Here's how the part is built. I have some questions about the finished solid (model axes, mm). A direction names the side the tool comes from. Give positions to 0.01 mm unless a question says otherwise; leave off trailing zeros. Loops run counter-clockwise (first coordinate to the right, second up) from the corner with the lowest first, then second, coordinate; pieces in that order, holes last. Notation, with made-up numbers: M -35,-31 L 10,-31 A21 ccw 10,-6 Z; hole C 64.5,-38.5 d11. An arc over 180 degrees is marked long. Answer as CSV lines item,"result". Start each with the question number.
Item 1: If I drill on line 1 along X through (y, z) = (2, 0); line 2 along X through (y, z) = (0.25, 0); line 3 along Y through (x, z) = (-20, 1.25), over which ranges is the centre line in solid material (lowest first)? Write a range as from..to.
Item 2: Will these pins go through, and if not, where does the flat tip stop? P1, Ø1, axis at y = 2.5, z = 0.5, coming from the -X side; P2, Ø1.5, axis at y = 1.5, z = 2.5, coming from the -X side; P3, Ø2.5, axis at x = -26.99, z = 0, coming from the -Y side; P4, Ø1.5, axis at x = -2, y = 1, coming from the -Z side.
Item 3: I want a section at A-A on y = 2.4. List the corners of the cut face in (x, z) for me, plus the area to 3 significant figures.
Item 4: I want a section at C-C on y = 0.45. List the corners of the cut face in (x, z) for me, plus the area to 3 significant figures.
Item 5: For faces 5 (the cylindrical face through (-28.45, 0.49, -0.33)), 6 (the flat face through (-14.2, 3, 2.4)), 7 (the flat face through (-1, 1, 0.2)), 8 (the flat face through (-18.88, 1.99, -2.69)), 9 (the flat face through (-1, 1, -0.2)), which set-ups out of +Z, -Z, +X, -X, +Y, -Y let a thin tool reach every point of the face, with its end or its side?
Item 6: I want a section at B-B on x = -26. List the corners of the cut face in (y, z) for me.
Item 7: I want a section at D-D on x = -21. List the corners of the cut face in (y, z) for me.
Item 8: If we mould it in two halves opening along Z, with no side actions, what happens to faces 1 (the flat face through (-17.23, 1.48, -3.3)), 2 (the flat face through (-18.716, 1.986, 2.675)), 3 (the cylindrical face through (-10.857, 1.986, -0.046)), 4 (the flat face through (-18, 0, 0))? For each: released by +Z, released by -Z, zero draft, split by the parting line, or undercut.
from build123d import *

# Parameters (mm, degrees)
SKETCH2_R           = 1.5
BOSS_EXTRUDE1_DEPTH = 1
BOSS_EXTRUDE2_DEPTH = 3
FILLET1_R           = 3


with BuildPart() as part:
    # Sketch2 → Boss-Extrude1 (new body)
    with BuildSketch(Plane(origin=(0, 0, 0), x_dir=(1, 0, 0), z_dir=(0, 1, 0))):
        with BuildLine():
            Line((-24.633695323, -3.234416395), (-12.961942578, -2.130426094))
            ThreePointArc((-12.961942578, -2.130426094), (-10.856533145, 0), (-12.961942578, 2.130426094))
            Line((-12.961942578, 2.130426094), (-24.633695323, 3.234416395))
            ThreePointArc((-24.633695323, 3.234416395), (-30.987107864, 0), (-24.633695323, -3.234416395))
        make_face()
        with Locations(Location((-26.987107864, 0, 0), (0, 0, 270))):
            Circle(SKETCH2_R, mode=Mode.SUBTRACT)
    extrude(amount=BOSS_EXTRUDE1_DEPTH)

    # Sketch2<3> → Boss-Extrude2 (add)
    with BuildSketch(Plane(origin=(0, 0, 0), x_dir=(1, 0, 0), z_dir=(0, 1, 0))):
        with BuildLine():
            Line((-7.749705802, -2.2), (-7.749705802, -0.2))
            Line((-7.749705802, -0.2), (2.851546862, -0.2))
            Line((2.851546862, -0.2), (2.851546862, 0.2))
            Line((2.851546862, 0.2), (-7.749705802, 0.2))
            Line((-7.749705802, 0.2), (-7.749705802, 2.2))
            Line((-7.749705802, 2.2), (-26.987107864, 4.428352964))
            ThreePointArc((-26.987107864, 4.428352964), (-31.487107864, -0.071647036), (-26.987107864, -4.571647036))
            Line((-26.987107864, -4.571647036), (-7.749705802, -2.2))
        make_face()
        with BuildLine():
            ThreePointArc((-24.633695323, -3.234416395), (-30.987107864, 0), (-24.633695323, 3.234416395))
            Line((-24.633695323, 3.234416395), (-12.961942578, 2.130426094))
            ThreePointArc((-12.961942578, 2.130426094), (-10.856533145, 0), (-12.961942578, -2.130426094))
            Line((-12.961942578, -2.130426094), (-24.633695323, -3.234416395))
        make_face(mode=Mode.SUBTRACT)
    extrude(amount=BOSS_EXTRUDE2_DEPTH)

    # Fillet1
    # the kernel refuses this fillet: 3 mm, written as the material it adds along each edge
    with BuildSketch(Plane(origin=(-7.749705802, 0, 0.2), x_dir=(0, 0, 1), z_dir=(0, 1, 0))) as fillet1_piece_1:
        with BuildLine():
            CenterArc((3, 2.828427125), FILLET1_R, 180, 70.528779366)
            Line((0, 2.828427125), (-0.06, 2.828427125))
            Line((-0.06, 2.828427125), (-0.06, 0))
            Line((-0.06, 0), (0, -0.06))
            ThreePointArc((0, -0.06), (1, -0.06), (1.98, -0.056568542))
            Line((1.98, -0.056568542), (2, 0))
        make_face()
    extrude(amount=3)
    with BuildSketch(Plane(origin=(-7.749705802, 0, -0.2), x_dir=(1, 0, 0), z_dir=(0, 1, 0))) as fillet1_piece_2:
        with BuildLine():
            CenterArc((2.828427125, 3), FILLET1_R, 199.471220634, 70.528779366)
            Line((0, 2), (-0.056568542, 1.98))
            ThreePointArc((-0.056568542, 1.98), (-0.06, 1), (-0.06, 0))
            Line((-0.06, 0), (0, -0.06))
            Line((0, -0.06), (2.828427125, -0.06))
            Line((2.828427125, -0.06), (2.828427125, 0))
        make_face()
    extrude(amount=3)


solid = part.part
Result:
1,line 1,"-31.49..-30.99, -10.86..2.85"
1,line 2,"-31.49..-28.49, -25.49..2.85"
1,line 3,"0..1"
2,P1,"x = -31.49"
2,P2,"x = -31.16"
2,P3,"through"
2,P4,"z = -0.2"
3,outline,"M -26.99,-4.43 L -7.75,-2.2 A3 cw -4.92,-0.2 L 2.85,-0.2 L 2.85,0.2 L -4.92,0.2 A3 cw -7.75,2.2 L -26.99,4.57 A4.5 ccw Z; hole M -24.63,-3.23 L -12.96,-2.13 A2.13 ccw -12.96,2.13 L -24.63,3.23 A4 ccw long Z"
3,area,"55.6 mm^2"
4,outline,"M -26.99,-4.43 L -7.75,-2.2 A3 cw -4.92,-0.2 L 2.85,-0.2 L 2.85,0.2 L -4.92,0.2 A3 cw -7.75,2.2 L -26.99,4.57 A4.5 ccw Z; hole C -26.99,0 d3"
4,area,"161 mm^2"
5,face 5,"+Y, -Y"
5,face 6,"+Z, -Z, +X, -X, +Y"
5,face 7,"+Z, +X, +Y, -Y"
5,face 8,"+Y"
5,face 9,"-Z, +X, +Y, -Y"
6,outline,"M 0,-4.31 L 3,-4.31 L 3,-3.88 L 1,-3.88 L 1,-1.13 L 0,-1.13 Z; M 0,1.13 L 1,1.13 L 1,3.88 L 3,3.88 L 3,4.45 L 0,4.45 Z"
7,outline,"M 0,-3.73 L 3,-3.73 L 3,-2.89 L 1,-2.89 L 1,2.89 L 3,2.89 L 3,3.83 L 0,3.83 Z"
8,face 1,"released by -Z"
8,face 2,"undercut"
8,face 3,"undercut"
8,face 4,"zero draft"
